Work out the finished part from the listing and answer in its coordinate system (mm). Face numbers are marked on the shaded views. A direction names the side the tool comes from. Give positions to 0.01 mm unless a question says otherwise; leave off trailing zeros. Loops run counter-clockwise (first coordinate to the right, second up) from the corner with the lowest first, then second, coordinate; pieces in that order, holes last. Notation, with made-up numbers: (13.5, 79) - (19.5, 79) arc R18 ccw to (19.5, 103) - close; hole circle Ø5 at (18.25, 22.5). An arc over 180 degrees is marked (long way). One line per item, written item: value.
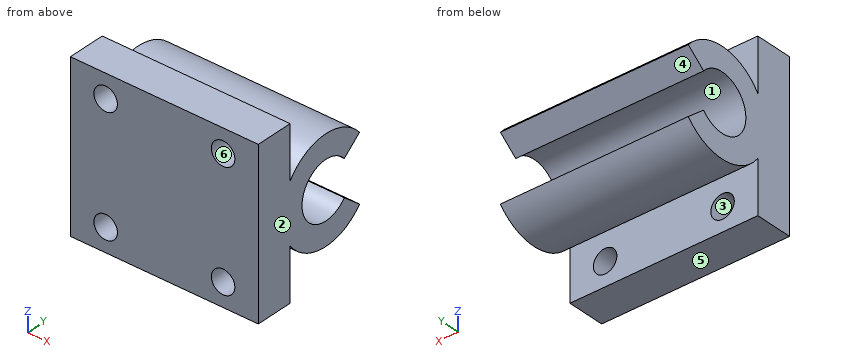
from build123d import *

# Parameters (mm, degrees)
EXTRUDE_1_DEPTH     = 20
CUT_EXTRUDE_1_REACH = 38.821
SKETCH_3_R          = 2.5


with BuildPart() as part:
    # Эскиз2 → Бобышка-Вытянуть1 (new, symmetric)
    with BuildSketch(Plane(origin=(0, 0, 0), x_dir=(0, 0, -1), z_dir=(1, 0, 0))):
        with BuildLine():
            Line((-3.818181818, 21.628335295), (-7, 25.485281374))
            ThreePointArc((-7, 25.485281374), (-10.991801936, 16.575394071), (-6.32455532, 8))
            Line((-6.32455532, 8), (-17.5, 8))
            Line((-17.5, 8), (-17.5, 0))
            Line((-17.5, 0), (17.5, 0))
            Line((17.5, 0), (17.5, 8))
            Line((17.5, 8), (6.32455532, 8))
            ThreePointArc((6.32455532, 8), (10.991801936, 16.575394071), (7, 25.485281374))
            Line((7, 25.485281374), (3.818181818, 21.628335295))
            ThreePointArc((3.818181818, 21.628335295), (0, 11), (-3.818181818, 21.628335295))
        make_face()
    extrude(amount=EXTRUDE_1_DEPTH, both=True)

    # Эскиз3 → Вырез-Вытянуть1 (cut, up to next)
    with BuildSketch(Plane.XZ, mode=Mode.PRIVATE) as cut_extrude_1_sk1:
        with Locations(Location((-12.5, 12.5, 0), (0, 0, 270))):
            Circle(SKETCH_3_R)
    cut_extrude_1_tool1 = extrude(cut_extrude_1_sk1.sketch, amount=-CUT_EXTRUDE_1_REACH, mode=Mode.PRIVATE) & part.part
    # Эскиз3 → Вырез-Вытянуть1 (cut, up to next)
    with BuildSketch(Plane.XZ, mode=Mode.PRIVATE) as cut_extrude_1_sk2:
        with Locations(Location((12.5, 12.5, 0), (0, 0, 270))):
            Circle(SKETCH_3_R)
    cut_extrude_1_tool2 = extrude(cut_extrude_1_sk2.sketch, amount=-CUT_EXTRUDE_1_REACH, mode=Mode.PRIVATE) & part.part
    # Эскиз3 → Вырез-Вытянуть1 (cut, up to next)
    with BuildSketch(Plane.XZ, mode=Mode.PRIVATE) as cut_extrude_1_sk3:
        with Locations(Location((-12.5, -12.5, 0), (0, 0, 270))):
            Circle(SKETCH_3_R)
    cut_extrude_1_tool3 = extrude(cut_extrude_1_sk3.sketch, amount=-CUT_EXTRUDE_1_REACH, mode=Mode.PRIVATE) & part.part
    # Эскиз3 → Вырез-Вытянуть1 (cut, up to next)
    with BuildSketch(Plane.XZ, mode=Mode.PRIVATE) as cut_extrude_1_sk4:
        with Locations(Location((12.5, -12.5, 0), (0, 0, 270))):
            Circle(SKETCH_3_R)
    cut_extrude_1_tool4 = extrude(cut_extrude_1_sk4.sketch, amount=-CUT_EXTRUDE_1_REACH, mode=Mode.PRIVATE) & part.part
    add(cut_extrude_1_tool1.solids().sort_by_distance((-12.5, 0, 12.5))[0], mode=Mode.SUBTRACT)
    add(cut_extrude_1_tool2.solids().sort_by_distance((12.5, 0, 12.5))[0], mode=Mode.SUBTRACT)
    add(cut_extrude_1_tool3.solids().sort_by_distance((-12.5, 0, -12.5))[0], mode=Mode.SUBTRACT)
    add(cut_extrude_1_tool4.solids().sort_by_distance((12.5, 0, -12.5))[0], mode=Mode.SUBTRACT)


solid = part.part
1. Section C-C (y = 5.5) is taken. Write down the section's boundary in (x, z), and give its area (3 significant figures).
Output:
outline: (-20, -17.5) - (20, -17.5) - (20, 17.5) - (-20, 17.5) - close; hole circle Ø5 at (-12.5, -12.5); hole circle Ø5 at (-12.5, 12.5); hole circle Ø5 at (12.5, -12.5); hole circle Ø5 at (12.5, 12.5)
area: 1,320 mm²
2. Section B-B (x = -12.5) is taken. Write down the section's boundary in (y, z).
Output:
outline: (0, -17.5) - (8, -17.5) - (8, -15) - (0, -15) - close; (0, -10) - (8, -10) - (8, -6.32) arc R11 ccw to (25.49, -7) - (21.63, -3.82) arc R6 cw (long way) to (21.63, 3.82) - (25.49, 7) arc R11 ccw to (8, 6.32) - (8, 10) - (0, 10) - close; (0, 15) - (8, 15) - (8, 17.5) - (0, 17.5) - close
3. Section D-D (x = 2) is taken. Write down the section's boundary in (y, z).
Output:
outline: (0, -17.5) - (8, -17.5) - (8, -6.32) arc R11 ccw to (25.49, -7) - (21.63, -3.82) arc R6 cw (long way) to (21.63, 3.82) - (25.49, 7) arc R11 ccw to (8, 6.32) - (8, 17.5) - (0, 17.5) - close
4. Find the intervals of material crossed by line 1 along X through (y, z) = (2, 12.5); line 2 along Z through (x, y) = (18.5, 16.5); line 3 along Y through (x, z) = (-0.5, -7.5), in increasing order.
Output:
line 1: x = -20 to -15, -10 to 10, 15 to 20
line 2: z = -10.99 to -5.98, 5.98 to 10.99
line 3: y = 0 to 8, 8.95 to 25.05
5. Section A-A (z = 12.5) is taken. Write down the section's boundary in (x, y).
Output:
outline: (-20, 0) - (-15, 0) - (-15, 8) - (-20, 8) - close; (-10, 0) - (10, 0) - (10, 8) - (-10, 8) - close; (15, 0) - (20, 0) - (20, 8) - (15, 8) - close
6. Flat-ended cylindrical pins translate along their axes: pin 1 Ø4 at (x, y) = (4, 17) entering from -Z; pin 2 Ø12 at (x, y) = (13.5, 14.5) entering from +Z; pin 3 Ø4 at (x, z) = (14.5, -4) entering from +Y. Find the tip coordinate at first contact, or state that the pin passes through.
Output:
pin 1: stops at z = -11
pin 2: stops at z = 11
pin 3: stops at y = 24.27
7. For the marked faces 4, 5 and 6, determine the directions among +Z, -Z, +X, -X, +Y, -Y from which every point of the face is accessible in a straight line to the end or side of a thin tool.
Output:
face 4: +X, -X, +Y
face 5: -Z, +X, -X, +Y, -Y
face 6: -Y
8. The mould has two halves that part along X. Classify the marked faces 1, 2 and 3: released by +X, released by -X, zero draft, split by the parting line, or undercut.
Output:
face 1: zero draft
face 2: released by +X
face 3: undercut
